Geometry check sheet. Reference: the model listing, model coordinates, mm. A direction names the side the tool comes from. Coordinates: 2 decimals unless noted, no trailing zeros. Loops run counter-clockwise (first coordinate to the right, second up) from the corner with the lowest first, then second, coordinate; pieces in that order, holes last.
from build123d import *

# Parameters (mm, degrees)
SKETCH_W        = 25
SKETCH_H        = 60
PAD_DEPTH       = 30
SKETCH001_W     = 20
SKETCH001_H     = 40
POCKET_DEPTH    = 27
SKETCH002_W     = 2.5
SKETCH002_H     = 30
POCKET001_DEPTH = 25
SKETCH003_W     = 2.5
SKETCH003_H     = 30
POCKET002_DEPTH = 25
SKETCH004_W     = 20
SKETCH004_H     = 24
POCKET003_DEPTH = 7
SKETCH005_W     = 20
SKETCH005_H     = 24
POCKET004_DEPTH = 7
SKETCH006_W     = 10
SKETCH006_H     = 7
POCKET005_DEPTH = 60.001
SKETCH007_R     = 1
POCKET006_DEPTH = 3
SKETCH008_R     = 1
POCKET007_DEPTH = 3


with BuildPart() as part:
    # Sketch → Pad (new body)
    with BuildSketch(Plane.XY):
        with Locations((12.5, 30)):
            Rectangle(SKETCH_W, SKETCH_H)
    extrude(amount=PAD_DEPTH)

    # Sketch001 (on Face6 of Pad) → Pocket (cut)
    with BuildSketch(Plane.XY.offset(30)):
        with Locations((12.5, 30)):
            Rectangle(SKETCH001_W, SKETCH001_H)
    extrude(amount=-POCKET_DEPTH, mode=Mode.SUBTRACT)

    # Sketch002 (on Face5 of Pocket) → Pocket001 (cut)
    with BuildSketch(Plane.XY.offset(30)):
        with Locations((1.25, 30)):
            Rectangle(SKETCH002_W, SKETCH002_H)
    extrude(amount=-POCKET001_DEPTH, mode=Mode.SUBTRACT)

    # Sketch003 (on Face5 of Pocket) → Pocket002 (cut)
    with BuildSketch(Plane.XY.offset(30)):
        with Locations((23.75, 30)):
            Rectangle(SKETCH003_W, SKETCH003_H)
    extrude(amount=-POCKET002_DEPTH, mode=Mode.SUBTRACT)

    # Sketch004 (on Face17 of Pocket002) → Pocket003 (cut)
    with BuildSketch(Plane.XZ.offset(-50)):
        with Locations((12.5, 15)):
            Rectangle(SKETCH004_W, SKETCH004_H)
    extrude(amount=-POCKET003_DEPTH, mode=Mode.SUBTRACT)

    # Sketch005 (on Face15 of Pocket002) → Pocket004 (cut)
    with BuildSketch(Plane(origin=(0, 10, 0), x_dir=(-1, 0, 0), z_dir=(0, 1, 0))):
        with Locations((-12.5, 15)):
            Rectangle(SKETCH005_W, SKETCH005_H)
    extrude(amount=-POCKET004_DEPTH, mode=Mode.SUBTRACT)

    # Sketch006 (on Face10 of Pocket004) → Pocket005 (cut, through all)
    with BuildSketch(Plane(origin=(0, 60, 0), x_dir=(-1, 0, 0), z_dir=(0, 1, 0))):
        with Locations((-12.5, 6.5)):
            Rectangle(SKETCH006_W, SKETCH006_H)
    extrude(amount=-POCKET005_DEPTH, mode=Mode.SUBTRACT)

    # Sketch007 (on Face4 of Pocket005) → Pocket006 (cut)
    with BuildSketch(Plane.XY.offset(30)):
        with Locations((6, 5)):
            Circle(SKETCH007_R)
        with Locations((19, 5)):
            Circle(SKETCH007_R)
    extrude(amount=-POCKET006_DEPTH, mode=Mode.SUBTRACT)

    # Sketch008 (on Face13 of Pocket005) → Pocket007 (cut)
    with BuildSketch(Plane.XY.offset(30)):
        with Locations((6, 55)):
            Circle(SKETCH008_R)
        with Locations((19, 55)):
            Circle(SKETCH008_R)
    extrude(amount=-POCKET007_DEPTH, mode=Mode.SUBTRACT)


solid = part.part
1) Material ranges on probe 1 along Y at (x, z) = (6, 28.5); probe 2 along Y at (x, z) = (21.75, 18.5); probe 3 along Z at (x, y) = (18.25, 3.5), recorded low to high.
Data:
probe 1: y = 0 to 4, 6 to 10, 50 to 54, 56 to 60
probe 2: y = 0 to 3, 57 to 60
probe 3: z = 0 to 3, 27 to 30
2) Section check C-C on z = 15.25. Record the cut outline in (x, y).
Data:
outline: (0, 0) - (25, 0) - (25, 15) - (22.5, 15) - (22.5, 3) - (2.5, 3) - (2.5, 15) - (0, 15) - close; (0, 45) - (2.5, 45) - (2.5, 57) - (22.5, 57) - (22.5, 45) - (25, 45) - (25, 60) - (0, 60) - close
3) Mould release check, pull along Z, two halves, no side actions. Record for faces 5 (the flat face through (13, 2, 10)), 6 (the flat face through (1, 45, 18)), 7 (the flat face through (12, 6, 30)): +Z half, -Z half, draft (parallel to the pull), parting line (faces both ways), or undercut.
Data:
face 5: undercut
face 6: draft
face 7: +Z half
4) Section check D-D on x = 23.75. Record the cut outline in (y, z).
Data:
outline: (0, 0) - (60, 0) - (60, 30) - (45, 30) - (45, 5) - (15, 5) - (15, 30) - (0, 30) - close
5) Section check A-A on y = 55. Record the cut outline in (x, z).
Data:
outline: (0, 0) - (25, 0) - (25, 30) - (20, 30) - (20, 27) - (22.5, 27) - (22.5, 3) - (2.5, 3) - (2.5, 27) - (5, 27) - (5, 30) - (0, 30) - close; (7, 27) - (18, 27) - (18, 30) - (7, 30) - close
6) Section check B-B on x = 11. Record the cut outline in (y, z).
Data:
outline: (0, 0) - (60, 0) - (60, 3) - (0, 3) - close; (0, 10) - (3, 10) - (3, 27) - (10, 27) - (10, 30) - (0, 30) - close; (50, 27) - (57, 27) - (57, 10) - (60, 10) - (60, 30) - (50, 30) - close
7) Depth check by flat-ended pin: pin 1 (3 mm diameter, centred on y = 49.5, z = 11.5, fed in from -X); pin 2 (1 mm diameter, centred on x = 8, y = 40.5, fed in from +Z); pin 3 (1.2 mm diameter, centred on x = 23, y = 24, fed in from +Z). Enter the tip coordinate at first touch or a pass-through.
Data:
pin 1: stops at x = 0
pin 2: stops at z = 3
pin 3: stops at z = 5
8) Access from +Z, -Z, +X, -X, +Y, -Y to the whole of each face (thin tool, end or side, straight path). Record for faces 1 (the flat face through (12, 50, 29)), 2 (the flat face through (1, 15, 18)), 3 (the flat face through (13, 59, 10)), 4 (the flat face through (13, 3, 18)).
Data:
face 1: +Z
face 2: +Z, +X, -X
face 3: +Y, -Y
face 4: none
